Design review of the part built by this model. Coordinates are the model's own, in mm. Give positions to 0.01 mm unless a question says otherwise; leave off trailing zeros. Loops run counter-clockwise (first coordinate to the right, second up) from the corner with the lowest first, then second, coordinate; pieces in that order, holes last. Notation, with made-up numbers: M 16,-32 L 23,-32 A13 cw 23,-14 Z; hole C 52,30.5 d6. An arc over 180 degrees is marked long. Use a Markdown table: item, result. Add a question column.
(1) Add section D-D, the plane y = 2. Give the boundary of the cut face in (x, z), then the cut area to 3 significant figures.
(2) Add section B-B, the plane z = -1.3. Give the boundary of the cut face in (x, y).
(3) Add section A-A, the plane y = -15. Give the boundary of the cut face in (x, z), then the cut area to 3 significant figures.
(4) Add section C-C, the plane x = 14. Give the boundary of the cut face in (y, z), then the cut area to 3 significant figures.
(5) For probe 1 along Y at (x, z) = (35, -1.5); probe 2 along Y at (x, z) = (-11, -2.75); probe 3 along X at (y, z) = (-16, -2.4), list the stretches that pass through material, from the lowest coordinate up.
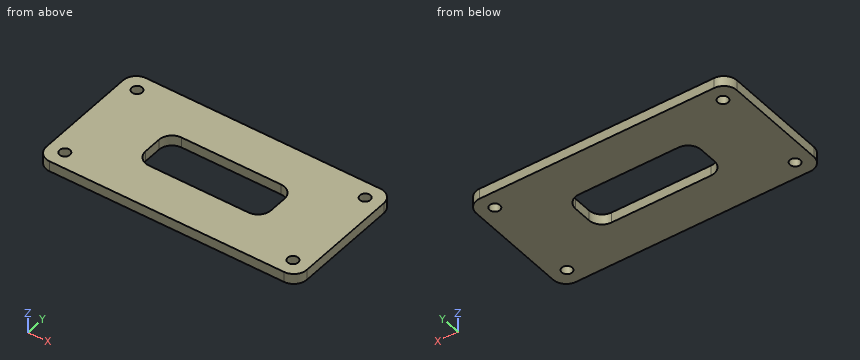
```python
from build123d import *

# Parameters (mm, degrees)
EXTRUDE_1_DEPTH     = 3.2
CUT_EXTRUDE_1_DEPTH = 3.2
SKETCH_3_R          = 1.6
CUT_EXTRUDE_2_DEPTH = 3.2


with BuildPart() as part:
    # 草图1 → 凸台-拉伸1 (new body)
    with BuildSketch(Plane.XY):
        with BuildLine():
            Line((-36, -20), (36, -20))
            ThreePointArc((36, -20), (38.828427125, -18.828427125), (40, -16))
            Line((40, -16), (40, 16))
            ThreePointArc((40, 16), (38.828427125, 18.828427125), (36, 20))
            Line((36, 20), (-36, 20))
            ThreePointArc((-36, 20), (-38.828427125, 18.828427125), (-40, 16))
            Line((-40, 16), (-40, -16))
            ThreePointArc((-40, -16), (-38.828427125, -18.828427125), (-36, -20))
        make_face()
    extrude(amount=-EXTRUDE_1_DEPTH)

    # 草图2 → 切除-拉伸1 (cut)
    with BuildSketch(Plane.XY):
        with BuildLine():
            Line((-15.25, -6.75), (15.25, -6.75))
            ThreePointArc((15.25, -6.75), (18.078427125, -5.578427125), (19.25, -2.75))
            Line((19.25, -2.75), (19.25, 2.75))
            ThreePointArc((19.25, 2.75), (18.078427125, 5.578427125), (15.25, 6.75))
            Line((15.25, 6.75), (-15.25, 6.75))
            ThreePointArc((-15.25, 6.75), (-18.078427125, 5.578427125), (-19.25, 2.75))
            Line((-19.25, 2.75), (-19.25, -2.75))
            ThreePointArc((-19.25, -2.75), (-18.078427125, -5.578427125), (-15.25, -6.75))
        make_face()
    extrude(amount=-CUT_EXTRUDE_1_DEPTH, mode=Mode.SUBTRACT)

    # 草图3 → 切除-拉伸2 (cut)
    with BuildSketch(Plane.XY):
        with Locations((-35, 15)):
            Circle(SKETCH_3_R)
        with Locations((35, 15)):
            Circle(SKETCH_3_R)
        with Locations((35, -15)):
            Circle(SKETCH_3_R)
        with Locations((-35, -15)):
            Circle(SKETCH_3_R)
    extrude(amount=-CUT_EXTRUDE_2_DEPTH, mode=Mode.SUBTRACT)


solid = part.part
```
Established:
| question | item | result |
|---|---|---|
| 1 | outline | M -40,-3.2 L -19.25,-3.2 L -19.25,0 L -40,0 Z; M 19.25,-3.2 L 40,-3.2 L 40,0 L 19.25,0 Z |
| 1 | area | 133 mm^2 |
| 2 | outline | M -40,-16 A4 ccw -36,-20 L 36,-20 A4 ccw 40,-16 L 40,16 A4 ccw 36,20 L -36,20 A4 ccw -40,16 Z; hole C -35,-15 d3.2; hole C -35,15 d3.2; hole M -19.25,-2.75 A4 ccw -15.25,-6.75 L 15.25,-6.75 A4 ccw 19.25,-2.75 L 19.25,2.75 A4 ccw 15.25,6.75 L -15.25,6.75 A4 ccw -19.25,2.75 Z; hole C 35,-15 d3.2; hole C 35,15 d3.2 |
| 3 | outline | M -40,-3.2 L -36.6,-3.2 L -36.6,0 L -40,0 Z; M -33.4,-3.2 L 33.4,-3.2 L 33.4,0 L -33.4,0 Z; M 36.6,-3.2 L 40,-3.2 L 40,0 L 36.6,0 Z |
| 3 | area | 236 mm^2 |
| 4 | outline | M -20,-3.2 L -6.75,-3.2 L -6.75,0 L -20,0 Z; M 6.75,-3.2 L 20,-3.2 L 20,0 L 6.75,0 Z |
| 4 | area | 84.8 mm^2 |
| 5 | probe 1 | -20 to -16.6, -13.4 to 13.4, 16.6 to 20 |
| 5 | probe 2 | -20 to -6.75, 6.75 to 20 |
| 5 | probe 3 | -40 to -36.25, -33.75 to 33.75, 36.25 to 40 |
